```python
from build123d import *

# Parameters (mm, degrees)
F0_W       = 22.7
F0_H       = 12.5
F1_DEPTH   = 22.5
F2_W       = 12.5
F2_H       = 2.5
F3_DEPTH   = 5
F4_W       = 12.5
F4_H       = 2.5
F5_DEPTH   = 5
F7_DEPTH   = 4.3
F8_R       = 2.15
F9_DEPTH   = 2.15
F10_R      = 2.5
F11_DEPTH  = 2.15
F12_W      = 3.9
F12_H      = 1.1
F13_DEPTH  = 0.1
F13_FACE_W = 3.9
F13_FACE_H = 1.1
F14_ANGLE  = 25
F15_W      = 3.9
F15_H      = 1.1
F16_DEPTH  = 10.6


with BuildPart() as f1:
    # F0 (on Top) → F1 (new body)
    with BuildSketch(Plane.XY):
        with Locations((6.858115, 5.973938)):
            Rectangle(F0_W, F0_H)
    extrude(amount=F1_DEPTH)

    # F2 (on face) → F3 (join)
    with BuildSketch(Plane(origin=(-4.491885, 0, 0), x_dir=(0, -1, 0), z_dir=(-1, 0, 0))):
        with Locations((-5.973938, 5.75)):
            Rectangle(F2_W, F2_H)
    extrude(amount=F3_DEPTH)

    # F4 (on face) → F5 (join)
    with BuildSketch(Plane.YZ.offset(18.208115)):
        with Locations((5.973938, 5.75)):
            Rectangle(F4_W, F4_H)
    extrude(amount=F5_DEPTH)

    # F6 (on face) → F7 (join)
    with BuildSketch(Plane(origin=(0, 0, 0), x_dir=(1, 0, 0), z_dir=(0, 0, -1))):
        with BuildLine():
            Line((5.608115, -8.873938), (6.315263, -8.873938))
            ThreePointArc((6.315263, -8.873938), (8.302885, -11.140399), (11.115966, -12.223938))
            Line((11.115966, -12.223938), (12.700264, -12.223938))
            ThreePointArc((12.700264, -12.223938), (16.634664, -10.139239), (18.208115, -5.973938))
            ThreePointArc((18.208115, -5.973938), (16.634664, -1.808637), (12.700264, 0.276062))
            Line((12.700264, 0.276062), (11.115966, 0.276062))
            ThreePointArc((11.115966, 0.276062), (8.302885, -0.807478), (6.315263, -3.073938))
            Line((6.315263, -3.073938), (5.608115, -3.073938))
            ThreePointArc((5.608115, -3.073938), (2.708115, -5.973938), (5.608115, -8.873938))
        make_face()
    extrude(amount=F7_DEPTH)

    # F8 (on face) → F9 (join)
    with BuildSketch(Plane(origin=(0, 0, -4.3), x_dir=(1, 0, 0), z_dir=(0, 0, -1))):
        with Locations((11.908115, -5.973938)):
            Circle(F8_R)
    extrude(amount=F9_DEPTH)

    # F10 (on face) → F11 (join)
    with BuildSketch(Plane(origin=(0, 0, -6.45), x_dir=(1, 0, 0), z_dir=(0, 0, -1))):
        with Locations((11.908115, -5.973938)):
            Circle(F10_R)
    extrude(amount=F11_DEPTH)

    # F12 (on face) → F13 (join)
    with BuildSketch(Plane.YZ.offset(18.208115)):
        with Locations((5.973938, 16.95)):
            Rectangle(F12_W, F12_H)
    extrude(amount=F13_DEPTH)

    # F13_face (on face) → F14 (revolve)
    with BuildSketch(Plane(origin=(18.308115, 5.973938, 16.95), x_dir=(0, 1, 0), z_dir=(1, 0, 0))):
        Rectangle(F13_FACE_W, F13_FACE_H)
    revolve(axis=Axis((18.208115, 5.973938, 22.5), (0, -1, 0)), revolution_arc=F14_ANGLE)

    # F15 (on face) → F16 (join)
    with BuildSketch(Plane(origin=(23.583096, 0, 10.996978), x_dir=(0, 1, 0), z_dir=(0.906308, 0, 0.422618))):
        with Locations((5.973938, 7.146843)):
            Rectangle(F15_W, F15_H)
    extrude(amount=F16_DEPTH)


solid = f1.part
```
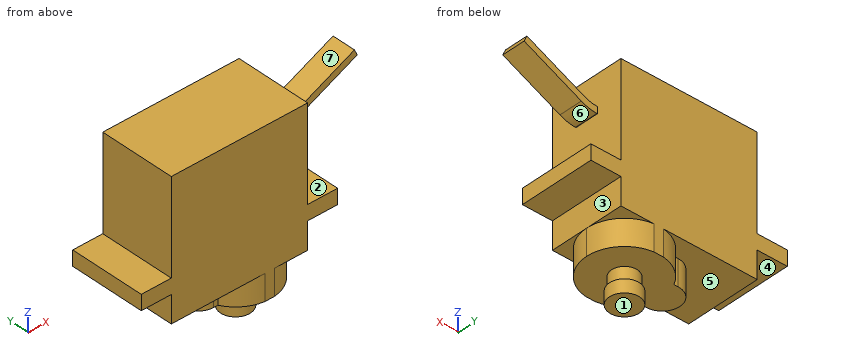
Source: CAD feature listing. Evaluate the final solid. Frame: model axes, mm. Face numbers are marked on the shaded views. A direction names the side the tool comes from. Round coordinates to 2 decimals unless told otherwise and drop trailing zeros. Write each loop counter-clockwise with the first axis right and the second up, starting at its lowest first coordinate (ties: lowest second). Pieces come first, ordered by that corner, then holes. Notation, with made-up numbers: M -13.5,74 L 2.5,74 A19 cw 2.5,89 Z; hole C 78.25,43 d10. An arc over 180 degrees is marked long. Use CSV: the item, a comma, the result in double quotes. Start each with the question number.
Q1. Line query: line 1 (Z direction, x = 4, y = 11.75); line 2 (X direction, y = 8.5, z = 15.5); line 3 (Z direction, x = -8, y = 10.25). Output: solid intervals per line, ascending. Write a range as from..to.
Q2. Cut plane D-D on x = 7.5. Output: boundary loops of the cut face in (y, z), plus the area to 3 significant figures.
Q3. First-contact query: P1, Ø4, axis at x = 21.5, y = 5.5, coming from the -Z side; P2, Ø6.5, axis at x = 26.5, z = 20, coming from the +Y side; P3, Ø3, axis at x = 6.5, z = -3, coming from the -Y side. Flat tips, straight axial feed; report the tip coordinate or a pass-through.
Q4. Cut plane C-C on z = -1.5. Output: boundary loops of the cut face in (x, y).
Q5. Cut plane B-B on x = 21.5. Output: boundary loops of the cut face in (y, z), plus the area to 3 significant figures.
Q6. Access query for the marked faces 4, 5, 6 and 7. Directions: +Z, -Z, +X, -X, +Y, -Y. A direction counts if a zero-diameter tool reaches every point of the face in a straight line with its end or side. Return the directions, or none.
Q7. Cut plane A-A on z = 19. Output: boundary loops of the cut face in (x, y), plus the area to 3 significant figures.
Q8. Pull-direction query (Z, two-part tool) for the marked faces 1, 2 and 3; classes: +Z half, -Z half, draft (parallel to the pull), parting line (faces both ways), or undercut.
Results found:
1,line 1,"0..22.5"
1,line 2,"-4.49..18.21"
1,line 3,"4.5..7"
2,outline,"M -0.28,0 L 1.47,0 L 1.47,-4.3 L 10.47,-4.3 L 10.47,0 L 12.22,0 L 12.22,22.5 L -0.28,22.5 Z"
2,area,"320 mm^2"
3,P1,"z = 4.5"
3,P2,"y = 7.92"
3,P3,"y = 1.03"
4,outline,"M 5.61,3.07 L 6.32,3.07 A6.3 ccw 11.12,-0.28 L 12.7,-0.28 A6.3 ccw 12.7,12.22 L 11.12,12.22 A6.3 ccw 6.32,8.87 L 5.61,8.87 A2.9 ccw Z"
5,outline,"M -0.28,4.5 L 12.22,4.5 L 12.22,7 L -0.28,7 Z; M 4.02,17.3 L 7.92,17.3 L 7.92,18.52 L 4.02,18.52 Z"
5,area,"36.0 mm^2"
6,face 4,"-Z, -X, +Y, -Y"
6,face 5,"-Z, -X"
6,face 6,"+X, +Y, -Y"
6,face 7,"+Z, +Y, -Y"
7,outline,"M -4.49,-0.28 L 18.21,-0.28 L 18.21,12.22 L -4.49,12.22 Z; M 22.53,4.02 L 25.14,4.02 L 25.14,7.92 L 22.53,7.92 Z"
7,area,"294 mm^2"
8,face 1,"-Z half"
8,face 2,"undercut"
8,face 3,"draft"
